Verification items for the finished model (mm, model axes). Face numbers are marked on the shaded views. A direction names the side the tool comes from. Give positions to 0.01 mm unless a question says otherwise; leave off trailing zeros. Order: outer loops, then holes, each group sorted by start corner. A loop starts at its lowest first (then second) coordinate and runs counter-clockwise, first axis right, second up. Notation, with made-up numbers: (29.5, -5) -> (54.5, -5) arc R25 cw to (54.5, 9) -> close; hole circle Ø8 at (38, -30.75). An arc over 180 degrees is marked (long way). Return JSON: item names as keys, results as strings. Group by question number.
(1) Cross-section at C-C on y = 12.75. Enter the section's corners in (x, z).
(2) Cross-section at D-D on x = 7.5. Enter the section's corners in (y, z), then the cut area to 3 significant figures.
(3) Thickness scan on line 1 along Y through (x, z) = (7.5, 21.75); line 2 along Z through (x, y) = (71, 4.75); line 3 along Y through (x, z) = (77.5, 27.2). Record the ranges inside material, lowest first.
(4) Cross-section at B-B on z = 27. Enter the section's corners in (x, y).
(5) Tool access check on the marked faces 1 and 2. Record the directions out of +Z, -Z, +X, -X, +Y, -Y that give a thin tool (end or side, any length) a straight path to the whole face; none if there is none.
(6) Release check for a two-part mould opening along Z. For the marked faces 3, 4 and 5 record: pulls with the +Z half, pulls with the -Z half, needs draft (parallel to the pull), parting line crosses it, or undercut.
(7) Cross-section at A-A on x = 21.5. Enter the section's corners in (y, z), then the cut area to 3 significant figures.
(8) Depth check by flat-ended pin: pin 1 Ø2 at (x, y) = (35, 5.5) entering from -Z; pin 2 Ø4 at (x, y) = (76.5, 4.5) entering from +Z. Enter the tip coordinate at first touch or a pass-through.
from build123d import *

# Parameters (mm, degrees)
CYLINDER002_R     = 3.3
CYLINDER002_DEPTH = 28
CYLINDER003_R     = 5
CYLINDER003_DEPTH = 6
CYLINDER_R        = 3.3
CYLINDER_DEPTH    = 28
CYLINDER001_R     = 5
CYLINDER001_DEPTH = 6
PAD_DEPTH         = 14


with BuildPart() as cilindro002:
    # Cylinder002 → Cylinder002 (new body)
    with BuildSketch(Plane.XY):
        Circle(CYLINDER002_R)
    extrude(amount=CYLINDER002_DEPTH)


with BuildPart() as obj1:
    # Cylinder003 → Cylinder003 (new body)
    with BuildSketch(Plane.XY.offset(26)):
        Circle(CYLINDER003_R)
    extrude(amount=CYLINDER003_DEPTH)

    # Fusion001: union Cilindro002
    add(cilindro002.part)


with BuildPart() as obj1_1:
    # Fusion001 placement: moved
    add(obj1.part.moved(Location((77.5, 7, 0))))


with BuildPart() as cilindro:
    # Cylinder → Cylinder (new body)
    with BuildSketch(Plane.XY):
        Circle(CYLINDER_R)
    extrude(amount=CYLINDER_DEPTH)


with BuildPart() as tornillos_m6:
    # Cylinder001 → Cylinder001 (new body)
    with BuildSketch(Plane.XY.offset(26)):
        Circle(CYLINDER001_R)
    extrude(amount=CYLINDER001_DEPTH)

    # Fusion: union Cilindro
    add(cilindro.part)


with BuildPart() as tornillos_m6_1:
    # Fusion placement: moved
    add(tornillos_m6.part.moved(Location((7.5, 7, 0))))

    # Fusion002: union obj1
    add(obj1_1.part)


with BuildPart() as obj2:
    # Sketch → Pad (new body)
    with BuildSketch(Plane.XZ):
        with BuildLine():
            Line((0, 0), (85, 0))
            Line((85, 0), (85, 17))
            Line((85, 17), (69.41608, 17))
            ThreePointArc((69.41608, 19), (57.5, 18), (69.41608, 17))
            Line((85, 19), (69.41608, 19))
            Line((85, 32), (85, 19))
            Line((0, 32), (85, 32))
            Line((0, 19), (0, 32))
            Line((0, 19), (15.58392, 19))
            ThreePointArc((15.58392, 17), (27.5, 18), (15.58392, 19))
            Line((0, 17), (15.58392, 17))
            Line((0, 0), (0, 17))
        make_face()
    extrude(amount=-PAD_DEPTH)

    # Cut: cut Tornillos_M6
    add(tornillos_m6_1.part, mode=Mode.SUBTRACT)


solid = obj2.part
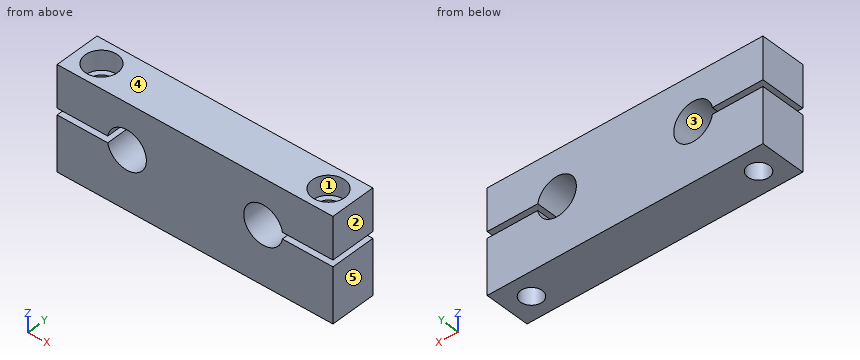
Verdict:
{
 "1": {"outline": "(0, 0) -> (85, 0) -> (85, 17) -> (69.42, 17) arc R6 cw (long way) to (69.42, 19) -> (85, 19) -> (85, 32) -> (0, 32) -> (0, 19) -> (15.58, 19) arc R6 cw (long way) to (15.58, 17) -> (0, 17) -> close"},
 "2": {"outline": "(0, 0) -> (3.7, 0) -> (3.7, 17) -> (0, 17) -> close; (0, 19) -> (3.7, 19) -> (3.7, 26) -> (2, 26) -> (2, 32) -> (0, 32) -> close; (10.3, 0) -> (14, 0) -> (14, 17) -> (10.3, 17) -> close; (10.3, 19) -> (14, 19) -> (14, 32) -> (12, 32) -> (12, 26) -> (10.3, 26) -> close", "area": "202 mm²"},
 "3": {"line 1": "0 to 3.7, 10.3 to 14", "line 2": "0 to 17, 19 to 32", "line 3": "0 to 2, 12 to 14"},
 "4": {"outline": "(0, 0) -> (85, 0) -> (85, 14) -> (0, 14) -> close; hole circle Ø10 at (7.5, 7); hole circle Ø10 at (77.5, 7)"},
 "5": {"face 1": "+Z", "face 2": "+Z, -Z, +X, +Y, -Y"},
 "6": {"face 3": "undercut", "face 4": "pulls with the +Z half", "face 5": "needs draft"},
 "7": {"outline": "(0, 0) -> (14, 0) -> (14, 12) -> (0, 12) -> close; (0, 24) -> (14, 24) -> (14, 32) -> (0, 32) -> close", "area": "280 mm²"},
 "8": {"pin 1": "z = 0", "pin 2": "z = 26"}
}
